Can you work these out from the model? Positions are in its coordinate system, mm. A direction names the side the tool comes from. Give positions to 0.01 mm unless a question says otherwise; leave off trailing zeros. Loops run counter-clockwise (first coordinate to the right, second up) from the corner with the lowest first, then second, coordinate; pieces in that order, holes last. Notation, with made-up numbers: M 63.25,80.5 L 100.25,80.5 A9 ccw 100.25,92.5 Z; hole C 6,74.25 d5. An arc over 180 degrees is marked long. Answer as a JSON object with one key per item and string values.
```python
from build123d import *

# Parameters (mm, degrees)
SKETCH1_R           = 15.25
SKETCH1_R_2         = 14.05
BOSS_EXTRUDE1_DEPTH = 5.2
CUT_EXTRUDE1_DEPTH  = 2
SKETCH4_R           = 17.05
SKETCH4_R_2         = 14.05
BOSS_EXTRUDE2_DEPTH = 12


with BuildPart() as part:
    # Sketch1 → Boss-Extrude1 (new body)
    with BuildSketch(Plane.XY):
        Circle(SKETCH1_R)
        Circle(SKETCH1_R_2, mode=Mode.SUBTRACT)
    extrude(amount=BOSS_EXTRUDE1_DEPTH)

    # Sketch2 → Cut-Extrude1 (cut)
    with BuildSketch(Plane.XY):
        Polygon((-0.75, 17.451253501), (0.75, 17.451253501), (0.75, 0.75), (21.876520237, 0.75), (21.876520237, -0.75), (0.75, -0.75), (0.75, -17.451253501), (-0.75, -17.451253501), (-0.75, -0.75), (-21.876520237, -0.75), (-21.876520237, 0.75), (-0.75, 0.75), align=None)
    extrude(amount=CUT_EXTRUDE1_DEPTH, mode=Mode.SUBTRACT)

    # Sketch4 → Boss-Extrude2 (add)
    with BuildSketch(Plane.XY.offset(5.2)):
        Circle(SKETCH4_R)
        Circle(SKETCH4_R_2, mode=Mode.SUBTRACT)
    extrude(amount=BOSS_EXTRUDE2_DEPTH)


solid = part.part
```
1) Will these pins go through, and if not, where does the flat tip stop? pin 1 Ø1.3 at (x, y) = (0, 14.5) entering from -Z; pin 2 Ø1.3 at (x, z) = (14.5, 1.5) entering from +Y; pin 3 Ø1 at (x, z) = (-14.5, 1) entering from -Y.
Answer list:
{"pin 1": "z = 2", "pin 2": "y = 6.38", "pin 3": "y = -6.05"}
2) Suppose I cut it at C-C, the plane z = 2.75. Write out the boundary of the cut face in (x, y), and give its area (3 significant figures).
Answer list:
{"outline": "C 0,0 d30.5; hole C 0,0 d28.1", "area": "110 mm^2"}
3) Suppose I cut it at A-A, the plane y = 0. Write out the boundary of the cut face in (x, z).
Answer list:
{"outline": "M -17.05,5.2 L -15.25,5.2 L -15.25,2 L -14.05,2 L -14.05,17.2 L -17.05,17.2 Z; M 14.05,2 L 15.25,2 L 15.25,5.2 L 17.05,5.2 L 17.05,17.2 L 14.05,17.2 Z"}
4) If we mould it in two halves opening along X, with no side actions, what happens to faces 1 (the flat face through (15, 0.75, 1)), 2 (the cylindrical face through (14.087, -5.841, 2.564)), 3 (the flat face through (0.75, -15, 1)), 4 (the cylindrical face through (12.98, -5.38, 8.48))? For each: +X half, -X half, draft (parallel to the pull), parting line (faces both ways), or undercut.
Answer list:
{"face 1": "draft", "face 2": "parting line", "face 3": "undercut", "face 4": "undercut"}
5) Please list where these lines run through material, in increasing order: line 1 along Y through (x, z) = (0, 8.25); line 2 along X through (y, z) = (0, 5). Write a range as from..to.
Answer list:
{"line 1": "-17.05..-14.05, 14.05..17.05", "line 2": "-15.25..-14.05, 14.05..15.25"}
6) For faces 5 (the flat face through (-15, -0.75, 1)), 6 (the cylindrical face through (-2.22, 16.905, 11.116)), 7 (the flat face through (-13, -9, 5.2)), 8 (the flat face through (-0.75, 15, 1)), 9 (the flat face through (10.1, -10.1, 0)), which set-ups out of +Z, -Z, +X, -X, +Y, -Y let a thin tool reach every point of the face, with its end or its side?
Answer list:
{"face 5": "-Z, +X, -X", "face 6": "+Z, -Z", "face 7": "-Z", "face 8": "-Z, +Y, -Y", "face 9": "-Z, +X, -X, +Y, -Y"}
7) Suppose I cut it at D-D, the plane z = 11.75. Write out the boundary of the cut face in (x, y), and give its area (3 significant figures).
Answer list:
{"outline": "C 0,0 d34.1; hole C 0,0 d28.1", "area": "293 mm^2"}
